Geometry check sheet. Reference: the model listing, model coordinates, mm. A direction names the side the tool comes from. Coordinates: 2 decimals unless noted, no trailing zeros. Write each loop counter-clockwise with the first axis right and the second up, starting at its lowest first coordinate (ties: lowest second). Pieces come first, ordered by that corner, then holes. Notation, with made-up numbers: (14, -4) -> (39, -4) arc R16 cw to (39, 3) -> close; hole circle Ø10 at (2, 21.25). An arc over 180 degrees is marked (long way). Answer as CSV lines item,"result".
```python
from build123d import *
from build123d.topology import SkipClean

# Parameters (mm, degrees)
SKETCH1_R              = 9.5
BOSS_EXTRUDE1_DEPTH    = 48
CUT_EXTRUDE1_DEPTH     = 62.48170459575759
BOSS_EXTRUDE2_START    = -2.5
SKETCH3_R              = 9.5
SKETCH3_R_2            = 2.4
BOSS_EXTRUDE2_DEPTH    = 2.5
SKETCH4_R              = 9.5
SKETCH4_R_2            = 4.2
BOSS_EXTRUDE3_DEPTH    = 7
SKETCH5_R              = 4.2
BOSS_EXTRUDE4_DEPTH    = 11
BOSS_EXTRUDE5_DEPTH    = 48
CUT_EXTRUDE2_START     = -48
CUT_EXTRUDE2_OUTLINE_R = 2.65
CUT_EXTRUDE2_DEPTH     = 48
CUT_EXTRUDE3_START     = -4.5
SKETCH8_R              = 9.5
CUT_EXTRUDE3_DEPTH     = 4.5
SKETCH9_R              = 6.067807638148196
CUT_EXTRUDE4_DEPTH     = 4.5
SKETCH10_R             = 9.5
BOSS_EXTRUDE6_DEPTH    = 4.5
SKETCH11_R             = 4.2
BOSS_EXTRUDE7_DEPTH    = 3.5
SKETCH12_R             = 2.4
BOSS_EXTRUDE8_DEPTH    = 2.5
CUT_EXTRUDE5_DEPTH     = 14.500000000000005
SKETCH15_R             = 3.436413098279149
BOSS_EXTRUDE9_DEPTH    = 10
BOSS_EXTRUDE10_DEPTH   = 0.5
SKETCH18_R             = 4.2
CUT_EXTRUDE8_DEPTH     = 0.5
CUT_EXTRUDE9_DEPTH     = 69.52919086053767
BOSS_EXTRUDE11_DEPTH   = 6.9999999999999964
CUT_EXTRUDE10_DEPTH    = 99.24586505293748
BOSS_EXTRUDE12_DEPTH   = 41.5
SKETCH25_R             = 4.2
CUT_EXTRUDE11_DEPTH    = 0.5
CUT_EXTRUDE12_DEPTH    = 99.24586505293753
CUT_EXTRUDE13_DEPTH    = 80.2290981899959


# Read off the part's stored shape, not the designer's step: Cut-Extrude2
with BuildPart() as part:
    # Sketch1 → Boss-Extrude1 (new body)
    with BuildSketch(Plane.XY):
        with BuildLine():
            Line((-12, 0), (-12, 30))
            Line((-12, 30), (12, 30))
            Line((12, 30), (12, 0))
            ThreePointArc((12, 0), (-2.2e-15, -12), (-12, 0))
        make_face()
        Circle(SKETCH1_R, mode=Mode.SUBTRACT)
    extrude(amount=-BOSS_EXTRUDE1_DEPTH)

    # Sketch2 → Cut-Extrude1 (cut, through all)
    with BuildSketch(Plane.ZY.offset(12)):
        Polygon((-6.999999999999999, -12), (-41, -12.000000000000004), (-41, 18), (-7.000000000000001, 18.000000000000004), align=None)
    extrude(amount=-CUT_EXTRUDE1_DEPTH, mode=Mode.SUBTRACT)

    # Sketch3 → Boss-Extrude2 (add)
    with BuildSketch(Plane(origin=(0, 0, -48), x_dir=(-1, 0, 0), z_dir=(0, 0, -1)).offset(BOSS_EXTRUDE2_START)):
        Circle(SKETCH3_R)
        Circle(SKETCH3_R_2, mode=Mode.SUBTRACT)
    extrude(amount=BOSS_EXTRUDE2_DEPTH)

    # Sketch4 → Boss-Extrude3 (add)
    with BuildSketch(Plane.XY):
        with Locations(Location((0, 0, 0), (0, 0, 180))):
            Circle(SKETCH4_R)
        Circle(SKETCH4_R_2, mode=Mode.SUBTRACT)
    extrude(amount=-BOSS_EXTRUDE3_DEPTH)

    # Sketch5 → Boss-Extrude4 (add)
    with BuildSketch(Plane.XY):
        Circle(SKETCH5_R)
    extrude(amount=-BOSS_EXTRUDE4_DEPTH)

    # Sketch6 → Boss-Extrude5 (add)
    with BuildSketch(Plane(origin=(0, 0, -48), x_dir=(-1, 0, 0), z_dir=(0, 0, -1))):
        Polygon((12, 30), (12, 18), (17.999999999999925, 18), (38.00000000000001, 18), (38.00000000000001, 30), align=None)
    extrude(amount=-BOSS_EXTRUDE5_DEPTH)

    # Cut-Extrude2 outline → Cut-Extrude2 (cut)
    with BuildSketch(Plane.XY.offset(CUT_EXTRUDE2_START)):
        Circle(CUT_EXTRUDE2_OUTLINE_R)
    extrude(amount=CUT_EXTRUDE2_DEPTH, mode=Mode.SUBTRACT)

    # Sketch8 → Cut-Extrude3 (cut)
    with BuildSketch(Plane(origin=(0, -4e-16, -7), x_dir=(-1, 0, 0), z_dir=(0, -6e-17, -1)).offset(CUT_EXTRUDE3_START)):
        Circle(SKETCH8_R)
    extrude(amount=CUT_EXTRUDE3_DEPTH, mode=Mode.SUBTRACT)


with BuildPart() as cut_extrude3_piece_1:
    # of the separate pieces the step leaves, piece 1, a body of its own (cut_extrude3_pieces)
    add(part.part.solids().sort_by_distance((-12, 0, 0))[0])

    # Sketch10 → Boss-Extrude6 (add)
    with BuildSketch(Plane.XY.offset(-45.5)):
        with Locations(Location((0, 0, 0), (0, 0, 90))):
            Circle(SKETCH10_R)
    extrude(amount=BOSS_EXTRUDE6_DEPTH)

    # Sketch11 → Boss-Extrude7 (add)
    with BuildSketch(Plane.XY.offset(-41)):
        with Locations(Location((0, 0, 0), (0, 0, 180))):
            Circle(SKETCH11_R)
    extrude(amount=BOSS_EXTRUDE7_DEPTH)

    # Sketch12 → Boss-Extrude8 (add)
    with BuildSketch(Plane(origin=(0, 0, -48), x_dir=(-1, 0, 0), z_dir=(0, 0, -1))):
        Circle(SKETCH12_R)
    extrude(amount=-BOSS_EXTRUDE8_DEPTH)

    # Sketch13 → Cut-Extrude5 (cut)
    with BuildSketch(Plane(origin=(0, 30, 0), x_dir=(1, 0, 0), z_dir=(0, 1, 0))):
        Polygon((12, 41), (-23.000000000000004, 41), (-22.999999999999996, 6.999999999999988), (12, 7.000000000000001), align=None)
    extrude(amount=-CUT_EXTRUDE5_DEPTH, mode=Mode.SUBTRACT)

    # Sketch15 → Boss-Extrude9 (add)
    with BuildSketch(Plane(origin=(0, 0, -48), x_dir=(-1, 0, 0), z_dir=(0, 0, -1))):
        Circle(SKETCH15_R)
    extrude(amount=-BOSS_EXTRUDE9_DEPTH)

    # Sketch16 → Boss-Extrude10 (add)
    with BuildSketch(Plane(origin=(0, 0, -48), x_dir=(-1, 0, 0), z_dir=(0, 0, -1))):
        Polygon((38.00000000000001, 30), (-12, 30), (-12, 18), (12, 18), (38.00000000000001, 18), align=None)
        with BuildLine():
            Line((-12, 0), (11.999999999999998, 0))
            ThreePointArc((11.999999999999998, 0), (-2.2e-15, -12), (-12, 0))
        make_face()
        with BuildLine():
            ThreePointArc((11.999999999999998, 0), (7.3e-16, 11.999999999999998), (-11.999999999999998, 1.47e-15))
            Line((-12, 0), (12, 0))
        make_face()
        with BuildLine():
            Line((12, 0), (-12, 0))
            ThreePointArc((-11.999999999999998, 1.47e-15), (-2.2e-15, -11.999999999999998), (11.999999999999998, -2.94e-15))
        make_face()
        with BuildLine():
            Line((12, 18), (-12, 18))
            Line((-12, 18), (-12, 0))
            ThreePointArc((-11.999999999999998, 1.47e-15), (7.3e-16, 11.999999999999998), (11.999999999999998, 0))
            Line((11.999999999999998, 0), (11.999999999999998, 18))
        make_face()
    extrude(amount=BOSS_EXTRUDE10_DEPTH)

    # Sketch18 → Cut-Extrude8 (cut)
    with SkipClean():  # the faces are left unmerged after this step: merging them gives an invalid solid
        with BuildSketch(Plane.XY.offset(-41)):
            with BuildLine():
                Line((12.000000000000004, 30), (-22.999999999999996, 30))
                Line((-22.999999999999996, 30), (-22.999999999999996, 18))
                Line((-22.999999999999996, 18), (-12.000000000000002, 18))
                Line((-12.000000000000002, 18), (-12.000000000000002, 0))
                ThreePointArc((-12, 1.47e-15), (-2.2e-15, -12), (12, -2.94e-15))
                Line((12, 0), (12, 30))
            make_face()
            Circle(SKETCH18_R, mode=Mode.SUBTRACT)
        extrude(amount=-CUT_EXTRUDE8_DEPTH, mode=Mode.SUBTRACT)

    # Sketch19 → Cut-Extrude9 (cut, through all)
    with SkipClean():  # the faces are left unmerged after this step: merging them gives an invalid solid
        with BuildSketch(Plane.XY):
            with BuildLine():
                ThreePointArc((11, -2.69e-15), (-2.02e-15, -11), (-11, 1.35e-15))
                Line((-11, 0), (-12.000000000000002, 0))
                ThreePointArc((-12.000000000000002, 0), (-7.3e-16, -12.000000000000002), (12.000000000000002, -1.47e-15))
                Line((12, 0), (12, 30))
                Line((12, 30), (11, 30))
                Line((11, 30), (11, 0))
            make_face()
        extrude(amount=-CUT_EXTRUDE9_DEPTH, mode=Mode.SUBTRACT)

    # Sketch21 → Boss-Extrude11 (add)
    with SkipClean():  # the faces are left unmerged after this step: merging them gives an invalid solid
        with BuildSketch(Plane.XY):
            with BuildLine():
                Line((-80, -11.000000000000007), (-2.02e-15, -11))
                ThreePointArc((-2.02e-15, -11), (-11, 7.951e-14), (1.5455e-13, 11))
                Line((-9.4e-16, 11), (-2e-17, 29.50098275984317))
                ThreePointArc((1.58451e-12, 29.500982759843026), (-43.87333050880174, 16.901328954446853), (-79.99999999999999, -11.000000000000014))
            make_face()
        boss_extrude11 = extrude(amount=-BOSS_EXTRUDE11_DEPTH)

    # Mirror2: Boss-Extrude11 across plane
    with SkipClean():  # the faces are left unmerged after this step: merging them gives an invalid solid
        add(boss_extrude11.mirror(Plane.XY.offset(-24.25)))

    # Sketch23 → Cut-Extrude10 (cut, through all)
    with SkipClean():  # the faces are left unmerged after this step: merging them gives an invalid solid
        with BuildSketch(Plane.XY):
            with BuildLine():
                Line((11, 30), (-38.00000000000001, 30))
                Line((-38.00000000000001, 30), (-38.00000000000001, 19.680026503546667))
                ThreePointArc((-38.000000000000014, 19.680026503546685), (-14.03748116807828, 27.39201372395351), (10.999999999999979, 30.00000000000003))
            make_face()
        extrude(amount=-CUT_EXTRUDE10_DEPTH, mode=Mode.SUBTRACT)

    # Sketch24 → Boss-Extrude12 (add)
    with BuildSketch(Plane.XY):
        with BuildLine():
            ThreePointArc((-23.00000000000003, 25.145323923706542), (-54.060518829682096, 11.110516861146493), (-80, -11))
            Line((-80, -11.000000000000007), (-75.95443157615205, -11.000000000000004))
            ThreePointArc((-75.95443157615205, -11.000000000000028), (-51.689916223605806, 9.057380529785846), (-22.999999999999986, 22.017084465179764))
            Line((-22.999999999999996, 22.017084465179774), (-23, 25.1453239237065))
        make_face()
    extrude(amount=-BOSS_EXTRUDE12_DEPTH)

    # Sketch25 → Cut-Extrude11 (cut)
    # profile 1 of 4: a face of its own
    with BuildSketch(Plane.XY.offset(-41.5)):
        with BuildLine():
            ThreePointArc((-34.29658362177963, 17.999999999999986), (-56.6966229233105, 5.756871837942555), (-75.95443157615205, -11.000000000000028))
            Line((-75.95443157615205, -11.000000000000007), (0, -11.000000000000007))
            ThreePointArc((-2.02e-15, -11), (-7.778174593052022, 7.778174593052023), (11, 0))
            Line((10.999999999999988, 0), (10.999999999999988, 26.999999999999993))
            ThreePointArc((10.999999999999988, 26.999999999999986), (-6.181599512464837, 25.74765282571859), (-22.999999999996817, 22.017084465180716))
            Line((-23, 22.01708446518151), (-23.000000000000004, 18))
            Line((-23.000000000000004, 18), (-34.29658362177963, 18.000000000000004))
        make_face()
    # profile 2 of 4: a face of its own
    with BuildSketch(Plane.XY.offset(-41.5)):
        with BuildLine():
            ThreePointArc((11, 0), (-7.778174593052022, 7.778174593052023), (-2.02e-15, -11))
            ThreePointArc((-2.02e-15, -11), (7.778174593052021, -7.778174593052024), (11, -2.69e-15))
        make_face()
        Circle(SKETCH25_R, mode=Mode.SUBTRACT)
    # profile 3 of 4: a face of its own
    with BuildSketch(Plane.XY.offset(-41.5)):
        with BuildLine():
            Line((-15.831452239273311, 26.999999999999996), (10.999999999999986, 26.999999999999996))
            Line((11, 26.999999999999996), (11, 30))
            ThreePointArc((10.999999999999591, 30), (-2.49932247622473, 29.24767054972125), (-15.83145223927318, 26.99999999999892))
        make_face()
    # profile 4 of 4: a face of its own
    with BuildSketch(Plane.XY.offset(-41.5)):
        with BuildLine():
            ThreePointArc((-15.83145223927318, 26.99999999999892), (-19.4298595333881, 26.127289318508147), (-22.99999999999981, 25.145323923705888))
            Line((-23, 25.14532392370651), (-23, 22.01708446518151))
            ThreePointArc((-22.999999999996817, 22.017084465180716), (-6.181599512464837, 25.74765282571859), (10.999999999999988, 26.999999999999986))
            Line((10.999999999999986, 26.999999999999996), (-15.831452239273311, 26.999999999999996))
        make_face()
    extrude(amount=-CUT_EXTRUDE11_DEPTH, mode=Mode.SUBTRACT)

    # Sketch26 → Cut-Extrude12 (cut, through all)
    with BuildSketch(Plane(origin=(0, 0, -48.5), x_dir=(-1, 0, 0), z_dir=(0, 0, -1))):
        with BuildLine():
            Line((54.999999999999986, 4.498697742403834), (54.99999999999999, -11))
            Line((55, -11), (70, -11))
            Line((70, -11), (73.20879972555869, -11.000000000000004))
            ThreePointArc((73.2087997255591, -10.99999999999882), (64.50313428378952, -2.7821940147532445), (55.00000000000103, 4.498697742404204))
        make_face()
        with BuildLine():
            Line((54.99999999999998, 10.508698660488534), (54.999999999999986, 4.498697742403834))
            ThreePointArc((55.00000000000103, 4.498697742404204), (64.50313428378952, -2.7821940147532445), (73.2087997255591, -10.99999999999882))
            Line((73.20879972555869, -11.000000000000004), (80, -11.00000000000001))
            ThreePointArc((80, -11), (68.23323816124723, 0.6066070293515935), (54.999999999999986, 10.508698660488534))
        make_face()
    extrude(amount=-CUT_EXTRUDE12_DEPTH, mode=Mode.SUBTRACT)

    # Sketch27 → Cut-Extrude13 (cut, through all)
    with BuildSketch(Plane(origin=(0, 0, -48.5), x_dir=(-1, 0, 0), z_dir=(0, 0, -1))):
        Polygon((54.999999999999986, -11.000000000000005), (44.999999999999986, -11.000000000000007), (44.999999999999986, -6.000000000000005), (54.999999999999986, -6.000000000000004), align=None)
    extrude(amount=-CUT_EXTRUDE13_DEPTH, mode=Mode.SUBTRACT)


with BuildPart() as cut_extrude3_piece_2:
    # of the separate pieces the step leaves, piece 2, a body of its own (cut_extrude3_pieces)
    add(part.part.solids().sort_by_distance((4.2, 0, -7))[0])

    # Sketch9 → Cut-Extrude4 (cut)
    with BuildSketch(Plane(origin=(0, 0, -11), x_dir=(-1, 0, 0), z_dir=(0, 0, -1))):
        Circle(SKETCH9_R)
    extrude(amount=-CUT_EXTRUDE4_DEPTH, mode=Mode.SUBTRACT)


solid = cut_extrude3_piece_1.part
```
Item 1: Cross-section at C-C, the plane z = -5. Record the cut outline in (x, y), plus the area to 3 significant figures.
Responses:
outline,"(-55, -6) -> (-45, -6) -> (-45, -11) -> (0, -11) arc R11 ccw to (11, 0) -> (11, 30) arc R121.49 ccw to (-55, 10.51) -> close; hole circle Ø19 at (0, 0)"
area,"1,930 mm2"
Item 2: Cross-section at A-A, the plane z = -40. Record the cut outline in (x, y).
Responses:
outline,"(-55, 6.92) arc R118.49 cw to (-34.3, 18) -> (-23, 18) -> (-23, 25.15) arc R121.49 ccw to (-55, 10.51) -> close; circle Ø8.4 at (0, 0)"
Item 3: Cross-section at D-D, the plane y = 15.5. Record the cut outline in (x, z).
Responses:
outline,"(-46.56, -48.5) -> (11, -48.5) -> (11, -42) -> (-39.92, -42) -> (-39.92, -7) -> (11, -7) -> (11, 0) -> (-46.56, 0) -> close"
Item 4: Set-up check for faces 1 (the flat face through (0, 0, -37.5)), 2 (the flat face through (-22, 10, -7)), 3 (the cylindrical face through (-4.38, -8.43, -4.72)): record each of +Z, -Z, +X, -X, +Y, -Y from which the full face is reachable in a straight line by a thin tool's end or side.
Responses:
face 1,"+X, -X, +Y, -Y"
face 2,"+X, -Y"
face 3,"none"
Item 5: Cross-section at B-B, the plane x = -17. Record the cut outline in (y, z).
Responses:
outline,"(-11, -48.5) -> (26.73, -48.5) -> (26.73, -42) -> (-11, -42) -> close; (-11, -7) -> (26.73, -7) -> (26.73, 0) -> (-11, 0) -> close"
Item 6: Release check for a two-part mould opening along X. For faces 4 (the flat face through (-2, -2, -2.5)), 5 (the flat face through (-45, -9, -4)), 6 (the flat face through (11, 15, -45)) record: +X half, -X half, draft (parallel to the pull), parting line (faces both ways), or undercut.
Responses:
face 4,"undercut"
face 5,"-X half"
face 6,"+X half"
Item 7: Depth check by flat-ended pin: pin 1 Ø6 at (x, y) = (0, 0) entering from +Z; pin 2 Ø6 at (x, z) = (-39, -20.5) entering from -Y; pin 3 Ø1.5 at (y, z) = (4.5, -27.5) entering from +X; pin 4 Ø2 at (x, z) = (-37.5, -16) entering from +Y. Enter the tip coordinate at first touch or a pass-through.
Responses:
pin 1,"stops at z = 0"
pin 2,"stops at y = 14.49"
pin 3,"passes through"
pin 4,"stops at y = 20.33"
Item 8: Thickness scan on probe 1 along Z at (x, y) = (-19, 10); probe 2 along Z at (x, y) = (3, 3.5); probe 3 along Y at (x, z) = (0, -3). Record the ranges inside material, lowest first.
Responses:
probe 1,"z = -48.5 to -42, -7 to 0"
probe 2,"z = -48.5 to -42, -2.5 to 0"
probe 3,"y = -11 to -9.5, 9.5 to 29.5"
